```python
from build123d import *

# Parameters (mm, degrees)
CHAMFER1_SIZE      = 0.5
CHAMFER2_SIZE      = 0.3
CUT_EXTRUDE1_DEPTH = 2.5
CHAMFER3_SIZE      = 0.3


with BuildPart() as part:
    # Sketch1 → Revolve1 (revolve)
    with BuildSketch(Plane.XY):
        Polygon((0, 0), (0, 2.75), (3, 2.75), (3, 1.49), (11, 1.49), (11, 0), align=None)
    revolve(axis=Axis((-88.705490849, 0, 0), (1, 0, 0)))

    # Chamfer1
    chamfer1_edges = [part.edges().sort_by_distance(p)[0] for p in [
        (11, -1.49, 0),
    ]]
    chamfer(chamfer1_edges, length=CHAMFER1_SIZE)

    # Chamfer2
    chamfer2_edges = [part.edges().sort_by_distance(p)[0] for p in [
        (0, -2.75, 0),
    ]]
    chamfer(chamfer2_edges, length=CHAMFER2_SIZE)

    # Sketch3 → Cut-Extrude1 (cut)
    with BuildSketch(Plane(origin=(0, 0, 0), x_dir=(0, 0, -1), z_dir=(1, 0, 0))):
        Polygon((-1.443375673, 0), (-0.721687836, -1.25), (0.721687836, -1.25), (1.443375673, 0), (0.721687836, 1.25), (-0.721687836, 1.25), align=None)
    extrude(amount=CUT_EXTRUDE1_DEPTH, mode=Mode.SUBTRACT)

    # Chamfer3
    chamfer3_edges = [part.edges().sort_by_distance(p)[0] for p in [
        (0, 0.625, 1.082531755),
        (0, -0.625, 1.082531755),
        (0, -1.25, 0),
        (0, -0.625, -1.082531755),
        (0, 0.625, -1.082531755),
        (0, 1.25, 0),
    ]]
    chamfer(chamfer3_edges, length=CHAMFER3_SIZE)


solid = part.part
```
Input: part model. Units: mm. Frame: model coordinates. A direction names the side the tool comes from. Coordinates: 2 decimals unless noted, no trailing zeros. Write each loop counter-clockwise with the first axis right and the second up, starting at its lowest first coordinate (ties: lowest second). Pieces come first, ordered by that corner, then holes.
1) Section A-A on z = 0. Output: boundary loops of the cut face in (x, y), and give its area (3 significant figures).
2) Set-up query: faces 4 (the flat face through (0.152, 0.71, 1.204)), 5 (the flat face through (0, -2, 0)). Return all of +Z, -Z, +X, -X, +Y, -Y with unobstructed straight access to the full face (end or side cutting, diameter ignored); none if empty.
3) Pin query (flat end, axial travel): pin 1 Ø2 at (x, y) = (6.5, -0.5) entering from +Z. Return the tip coordinate at first contact, or that it passes through.
4) Mould query, pull axis Y, two halves, no side actions, for faces 1 (the flat face through (0.152, -0.71, -1.204)), 2 (the flat face through (3, 1.2, -1.2)), 3 (the cylindrical face through (6.802, -0.194, 1.477)). Classes: pulls with the +Y half, pulls with the -Y half, needs draft (parallel to the pull), parting line crosses it, or undercut.
5) Section B-B on x = 7.75. Output: boundary loops of the cut face in (y, z), and give its area (3 significant figures).
6) Material intervals for line 1 along X through (y, z) = (1.25, 1.4); line 2 along X through (y, z) = (0.45, 0.6); line 3 along Y through (x, z) = (6, 0.05), sorted ascending.
Check result:
1. outline: (0, -2.45) - (0.3, -2.75) - (3, -2.75) - (3, -1.49) - (10.5, -1.49) - (11, -0.99) - (11, 0.99) - (10.5, 1.49) - (3, 1.49) - (3, 2.75) - (0.3, 2.75) - (0, 2.45) - (0, 1.55) - (0.3, 1.25) - (2.5, 1.25) - (2.5, -1.25) - (0.3, -1.25) - (0, -1.55) - close
1. area: 33.7 mm2
2. face 4: -X
2. face 5: +Z, -Z, -X, +Y, -Y
3. pin 1: stops at z = 1.49
4. face 1: undercut
4. face 2: needs draft
4. face 3: parting line crosses it
5. outline: circle Ø2.98 at (0, 0)
5. area: 6.97 mm2
6. line 1: x = 0 to 3
6. line 2: x = 2.5 to 11
6. line 3: y = -1.49 to 1.49
